```python
from build123d import *

# Parameters (mm, degrees)
SKETCH_1_R          = 1.358928477
SKETCH_1_R_2        = 1.599915794
SKETCH_1_R_3        = 1.649913162
SKETCH_1_W          = 3.996376927
SKETCH_1_H          = 6.806421868
SKETCH_1_H_2        = 6.790704991
SKETCH_1_W_2        = 4.032106697
SKETCH_1_W_3        = 10.92790885
SKETCH_1_H_3        = 3.891970495
SKETCH_1_W_4        = 13.80275679
SKETCH_1_W_5        = 2.328877428
SKETCH_1_H_4        = 1.692910899
SKETCH_1_W_6        = 2.328877427
SKETCH_1_H_5        = 1.6929109
SKETCH_1_W_7        = 24.700449722
SKETCH_1_H_6        = 13.915746322
EXTRUDE_1_DEPTH     = 3
SKETCH_2_R          = 1.6
CUT_EXTRUDE_1_DEPTH = 67.261211836


with BuildPart() as part:
    # 草图1 → 凸台-拉伸1 (new body)
    with BuildSketch(Plane(origin=(0, 0, 0), x_dir=(-1, 0, 0), z_dir=(0, 0, -1))):
        with BuildLine():
            Line((-56.997000158, -27.962959634), (-2.999842114, -27.962959634))
            ThreePointArc((-2.999842114, -27.962959634), (-0.878633413, -27.084326221), (0, -24.96311752))
            Line((0, -24.96311752), (0, 14.034849413))
            ThreePointArc((0, 14.034849413), (-0.693847958, 15.953558265), (-2.454424946, 16.984692259))
            Line((-2.454424946, 16.984692259), (-50.77996637, 25.919941108))
            Line((-50.77996637, 25.919941108), (-51.260080297, 25.919941108))
            ThreePointArc((-51.260080297, 25.919941108), (-53.255311763, 25.386759089), (-54.718604462, 23.929362046))
            Line((-54.718604462, 23.929362046), (-59.996842271, 14.843746718))
            Line((-59.996842271, 14.843746718), (-59.996842271, -24.96311752))
            ThreePointArc((-59.996842271, -24.96311752), (-59.118208859, -27.084326221), (-56.997000158, -27.962959634))
        make_face()
        with Locations(Location((-55.497079101, -15.463517499, 0), (0, 0, 180))):
            Circle(SKETCH_1_R, mode=Mode.SUBTRACT)
        with Locations(Location((-4.49976317, -15.463517499, 0), (0, 0, 180))):
            Circle(SKETCH_1_R, mode=Mode.SUBTRACT)
        with Locations(Location((-20.497921162, -4.53509268, 0), (0, 0, 180))):
            Circle(SKETCH_1_R_2, mode=Mode.SUBTRACT)
        with Locations(Location((-20.497921162, 14.46490732, 0), (0, 0, 180))):
            Circle(SKETCH_1_R_2, mode=Mode.SUBTRACT)
        with Locations(Location((-51.248302721, 21.868517657, 0), (0, 0, 180))):
            Circle(SKETCH_1_R_3, mode=Mode.SUBTRACT)
        with Locations((-4.436721131, -9.025383771)):
            Rectangle(SKETCH_1_W, SKETCH_1_H, mode=Mode.SUBTRACT)
        with Locations((-4.436721131, -22.000344001)):
            Rectangle(SKETCH_1_W, SKETCH_1_H_2, mode=Mode.SUBTRACT)
        with Locations((-55.302485972, -22.000344001)):
            Rectangle(SKETCH_1_W_2, SKETCH_1_H_2, mode=Mode.SUBTRACT)
        with Locations((-55.302485972, -9.025383771)):
            Rectangle(SKETCH_1_W_2, SKETCH_1_H, mode=Mode.SUBTRACT)
        with Locations((-12.771799921, -23.449711249)):
            Rectangle(SKETCH_1_W_3, SKETCH_1_H_3, mode=Mode.SUBTRACT)
        with Locations((-45.760922572, -23.449711249)):
            Rectangle(SKETCH_1_W_4, SKETCH_1_H_3, mode=Mode.SUBTRACT)
        with Locations((-47.892979317, 7.443776854)):
            Rectangle(SKETCH_1_W_5, SKETCH_1_H_4, mode=Mode.SUBTRACT)
        with Locations((-47.840982053, 2.205052576)):
            Rectangle(SKETCH_1_W_6, SKETCH_1_H_5, mode=Mode.SUBTRACT)
        with Locations((-20.421644705, 5.082457397)):
            Rectangle(SKETCH_1_W_7, SKETCH_1_H_6, mode=Mode.SUBTRACT)
    extrude(amount=-EXTRUDE_1_DEPTH)

    # 草图2 → 切除-拉伸1 (cut, through all)
    with BuildSketch(Plane.XY.offset(3)):
        with Locations((55.497079101, -15.463517499)):
            Circle(SKETCH_2_R)
        with Locations((4.49976317, -15.463517499)):
            Circle(SKETCH_2_R)
    extrude(amount=-CUT_EXTRUDE_1_DEPTH, mode=Mode.SUBTRACT)


solid = part.part
```
For this review, take the finished solid that the model builds, in its own axes (mm). A direction names the side the tool comes from. Round coordinates to 2 decimals unless told otherwise and drop trailing zeros. Order: outer loops, then holes, each group sorted by start corner. A loop starts at its lowest first (then second) coordinate and runs counter-clockwise, first axis right, second up. Notation, with made-up numbers: (25, -17.75) -> (65, -17.75) arc R9 cw to (65, -0.75) -> close; hole circle Ø1 at (5, 7). An arc over 180 degrees is marked (long way). Use a Markdown table: item, result.
Item 1: For pin 1 (1.2 mm diameter, centred on x = 48, z = 1.5, fed in from +Y); pin 2 (8 mm diameter, centred on x = 16.5, y = 1, fed in from -Z), all flat-tipped, find the tip position at first contact; note any pin that passes through.
Resolved:
| item | result |
|---|---|
| pin 1 | stops at y = 25.52 |
| pin 2 | stops at z = 0 |
Item 2: Draft analysis for pull direction X (two halves, no side actions). For faces 1 (the flat face through (30, -27.963, 1)), 2 (the flat face through (26.28, 21.39, 1.48)), 3 (the flat face through (55, -5.622, 1)), 4 (the flat face through (2.439, -22, 1)), state which applies: +X half, -X half, draft (parallel to the pull), parting line (faces both ways), or undercut.
Resolved:
| item | result |
|---|---|
| face 1 | draft |
| face 2 | -X half |
| face 3 | undercut |
| face 4 | undercut |
Item 3: For line 1 along X through (y, z) = (-10.5, 0.2); line 2 along X through (y, z) = (-24.5, 0.2); line 3 along Y through (x, z) = (51, 0.3), list the stretches that pass through material, from the lowest coordinate up. Write a range as [from, to].
Resolved:
| item | result |
|---|---|
| line 1 | x = [0, 2.44], [6.43, 53.29], [57.32, 60] |
| line 2 | x = [0, 2.44], [6.43, 7.31], [18.24, 38.86], [52.66, 53.29], [57.32, 60] |
| line 3 | y = [-27.96, -25.4], [-21.5, 20.24], [23.5, 25.92] |
Item 4: Take a section at C-C (y = 0). State the section outline as (x, z) points, plus the area to 3 significant figures.
Resolved:
| item | result |
|---|---|
| outline | (0, 0) -> (8.07, 0) -> (8.07, 3) -> (0, 3) -> close; (32.77, 0) -> (60, 0) -> (60, 3) -> (32.77, 3) -> close |
| area | 106 mm² |
Item 5: Take a section at D-D (x = 48). State the section outline as (y, z) points.
Resolved:
| item | result |
|---|---|
| outline | (-27.96, 0) -> (-25.4, 0) -> (-25.4, 3) -> (-27.96, 3) -> close; (-21.5, 0) -> (1.36, 0) -> (1.36, 3) -> (-21.5, 3) -> close; (3.05, 0) -> (6.6, 0) -> (6.6, 3) -> (3.05, 3) -> close; (8.29, 0) -> (25.41, 0) -> (25.41, 3) -> (8.29, 3) -> close |
Item 6: Take a section at A-A (y = -8.5). State the section outline as (x, z) points.
Resolved:
| item | result |
|---|---|
| outline | (0, 0) -> (2.44, 0) -> (2.44, 3) -> (0, 3) -> close; (6.43, 0) -> (53.29, 0) -> (53.29, 3) -> (6.43, 3) -> close; (57.32, 0) -> (60, 0) -> (60, 3) -> (57.32, 3) -> close |
Item 7: Machinability: for faces 5 (the cylindrical face through (0.902, -27.108, 1.479)), 6 (the flat face through (13, -21.504, 1)), which of the approach directions +Z, -Z, +X, -X, +Y, -Y give a long, thin tool a straight path to every point of the face, cutting with its end or side? Answer none if there is none.
Resolved:
| item | result |
|---|---|
| face 5 | +Z, -Z, -X, -Y |
| face 6 | +Z, -Z |
Item 8: Take a section at B-B (x = 27). State the section outline as (y, z) points, plus the area to 3 significant figures.
Resolved:
| item | result |
|---|---|
| outline | (-27.96, 0) -> (-1.88, 0) -> (-1.88, 3) -> (-27.96, 3) -> close; (12.04, 0) -> (21.52, 0) -> (21.52, 3) -> (12.04, 3) -> close |
| area | 107 mm² |
